Geometry: see drawing. Coordinates: mm, zero at the bounding-box minimum. Coordinates: 2 decimals unless noted, no trailing zeros. Write each loop counter-clockwise with the first axis right and the second up, starting at its lowest first coordinate (ties: lowest second). Pieces come first, ordered by that corner, then holes. Notation, with made-up numbers: (-11.5, 24) - (12.5, 24) arc R24 cw to (12.5, 50) - close; hole circle Ø2 at (86.25, -35). An arc over 180 degrees is marked (long way). Use a Markdown table: item, result. Add a question column.
Q1. Material intervals for probe 1 along X at (y, z) = (12.75, 58.5) (1 decimal); probe 2 along X at (y, z) = (1.5, 19.05), sorted ascending. Write a range as from..to.
Q2. Section query D-D (x = 12.7). Give the number of separate pieces and of enclosed holes in the cut face.
Q3. Section query A-A (y = 10.25). Return the cut outline in (x, z) (1 decimal).
Q4. Section query C-C (z = 19.05). Return the cut outline in (x, y) (1 decimal), then the cut area to 3 significant figures.
Q5. Section query B-B (z = 89). Return the cut outline in (x, y) (1 decimal).
Q6. Pin query (flat end, axial travel): P1, Ø11, axis at x = 12.7, z = 6.35, coming from the +Y side. Return the tip coordinate at first contact, or that it passes through.
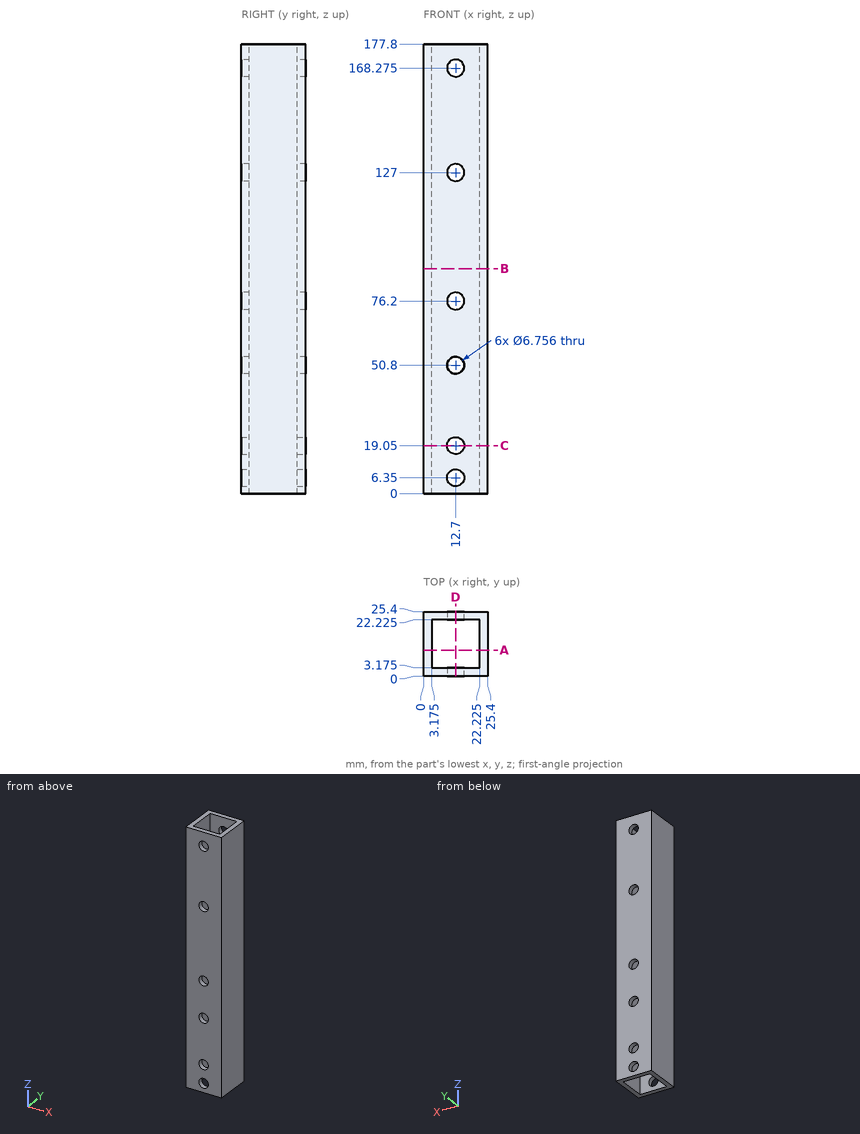
Values follow:
| question | item | result |
|---|---|---|
| 1 | probe 1 | 0..3.2, 22.2..25.4 |
| 1 | probe 2 | 0..9.32, 16.08..25.4 |
| 2 | separate pieces | 14 |
| 2 | enclosed holes | 0 |
| 3 | outline | (0, 0) - (3.2, 0) - (3.2, 177.8) - (0, 177.8) - close; (22.2, 0) - (25.4, 0) - (25.4, 177.8) - (22.2, 177.8) - close |
| 4 | outline | (0, 0) - (9.3, 0) - (9.3, 3.2) - (3.2, 3.2) - (3.2, 22.2) - (9.3, 22.2) - (9.3, 25.4) - (0, 25.4) - close; (16.1, 0) - (25.4, 0) - (25.4, 25.4) - (16.1, 25.4) - (16.1, 22.2) - (22.2, 22.2) - (22.2, 3.2) - (16.1, 3.2) - close |
| 4 | area | 239 mm2 |
| 5 | outline | (0, 0) - (25.4, 0) - (25.4, 25.4) - (0, 25.4) - close; hole (3.2, 3.2) - (22.2, 3.2) - (22.2, 22.2) - (3.2, 22.2) - close |
| 6 | P1 | y = 25.4 |
